The model under review builds one solid part; all positions refer to its coordinate system, in mm. A direction names the side the tool comes from. Round coordinates to 2 decimals unless told otherwise and drop trailing zeros. Write each loop counter-clockwise with the first axis right and the second up, starting at its lowest first coordinate (ties: lowest second). Pieces come first, ordered by that corner, then holes. Notation, with made-up numbers: (-19.75, -25.75) -> (24.25, -25.75) arc R23 ccw to (24.25, 4.25) -> close; hole circle Ø7 at (53.5, -12). An arc over 180 degrees is marked (long way). Return JSON: item names as keys, results as strings. Group by question number.
1. Take a section at A-A, the plane y = 0. Write out the cut boundary in (x, z) (3 decimals), then the cut area to 3 significant figures.
2. Take a section at B-B, the plane z = 127.5. Write out the cut boundary in (x, y) (3 decimals).
3. Mouldability with a two-part tool opening along Y and no side actions: class faces 4 (the flat face through (4, 16, 25.4)), 5 (the flat face through (7, -3, 0)), 6 (the cylindrical face through (15.12, 11.59, 6.62)) as pulls with the +Y half, pulls with the -Y half, needs draft (parallel to the pull), parting line crosses it, or undercut.
4. Tool access review of faces 1 (the cylindrical face through (3.441, 15.497, -6.261)), 2 (the cylindrical face through (-0.186, 15.878, 381.356)), 3 (the flat face through (7, -3, 609.6)): name each direction out of +Z, -Z, +X, -X, +Y, -Y from which nothing blocks a thin tool from reaching the whole face with its end or side.
5. Clearance check with flat-ended pins moving along their axes: P1, Ø1.5, axis at y = 2.5, z = 88.5, coming from the +X side; P2, Ø1.5, axis at y = 14, z = 294, coming from the -X side; P3, Ø10.5, axis at x = -5.5, y = 19, coming from the +Z side; P4, Ø4, axis at x = -2, z = 404, coming from the +Y side. State where each tip first meets the part, or that it passes through.
6. For line 1 along Y through (x, z) = (1, 389.5); line 2 along Y through (x, z) = (0, 370.5) (3 decimals); line 3 along X through (y, z) = (1, 532), list the stretches that pass through material, from the lowest coordinate up. Write a range as from..to.
Autodesk Inventor part; units mm, degrees
ref_plane "YZ Plane" through (0, 0, 0) normal (1, 0, 0) x (0, 1, 0)
ref_plane "XZ Plane" through (0, 0, 0) normal (0, 1, 0) x (-1, 0, 0)
ref_plane "XY Plane" through (0, 0, 0) normal (0, 0, 1) x (1, 0, 0)
sketch "Sketch1" plane through (0, 0, 0) normal (0, 0, 1) x (1, 0, 0)
  circle A0 centre (0, 0) radius 6.985
  circle A1 centre (0, 0) radius 15.875
  dimension "d0" = 13.97
  dimension "d1" = 31.75
extrude "Extrusion1" add sketch "Sketch1" along normal blind 609.6
ref_plane "Work Plane1" through (0, 0, 25.4) normal (0, 0, -1) x (-1, 0, 0)
sketch "Sketch2" plane through (0, 0, 25.4) normal (0, 0, -1) x (-1, 0, 0)
  circle A0 centre (0, 0) radius 19.05
  circle A1 centre (0, 0) radius 15.875
  dimension "d5" = 38.1
extrude "Extrusion2" add sketch "Sketch2" along normal blind 38.1
ref_plane "Work Plane2" through (0, 0, 406.4) normal (0, 0, -1) x (-1, 0, 0)
sketch "Sketch4" plane through (0, 0, 406.4) normal (0, 0, -1) x (-1, 0, 0)
  circle A0 centre (0, 0) radius 15.875
  arc A1 (-5.5104, 25.3806) -> (5.5104, 25.3806) centre (0, 22.225) ccw
  line L0 (8.9871, 25.3806) -> (5.5104, 25.3806)
  line L1 (-5.5104, 25.3806) -> (-8.9871, 25.3806)
  arc A2 (-8.9871, 25.3806) -> (-5.8921, 14.7411) centre (0, 22.225) ccw
  arc A3 (5.8921, 14.7411) -> (8.9871, 25.3806) centre (0, 22.225) ccw
  line L2 (5.8921, 14.7411) -> (-5.8921, 14.7411)
  point P0 (0, 15.875)
extrude "Extrusion3" add sketch "Sketch4" along normal blind 50.8 contours A0 A1 L0 A3 | A2 L1 A1 A0
ref_plane "Work Plane4" through (0, 0, 228.6) normal (0, 0, -1) x (-1, 0, 0)
sketch "Sketch6" plane through (0, 0, 228.6) normal (0, 0, -1) x (-1, 0, 0)
  circle A0 centre (0, 0) radius 15.875
  circle A1 centre (0, 0) radius 28.575
  circle A2 centre (0, 0) radius 22.225
  circle A3 centre (-22.225, 0) radius 6.35
  dimension "d23" = 44.45
  dimension "d22" = 57.15
  dimension "d24" = 12.7
properties part number "Blow Dart"
Output:
{
 "1": {"outline": "(-19.05, -12.7) -> (-15.875, -12.7) -> (-15.875, 0) -> (-6.985, 0) -> (-6.985, 609.6) -> (-15.875, 609.6) -> (-15.875, 25.4) -> (-19.05, 25.4) -> close; (6.985, 0) -> (15.875, 0) -> (15.875, -12.7) -> (19.05, -12.7) -> (19.05, 25.4) -> (15.875, 25.4) -> (15.875, 609.6) -> (6.985, 609.6) -> close", "area": "11,100 mm^2"},
 "2": {"outline": "circle Ø31.75 at (0, 0); hole circle Ø13.97 at (0, 0)"},
 "3": {"face 4": "needs draft", "face 5": "undercut", "face 6": "parting line crosses it"},
 "4": {"face 1": "-Z", "face 2": "+Z", "face 3": "+Z, +X, -X, +Y, -Y"},
 "5": {"P1": "stops at x = 15.78", "P2": "stops at x = -8.74", "P3": "stops at z = 609.6", "P4": "stops at y = 17.29"},
 "6": {"line 1": "y = -15.84..-6.91, 6.91..15.95", "line 2": "y = -15.875..-6.985, 6.985..15.875", "line 3": "x = -15.84..-6.91, 6.91..15.84"}
}
